Work out the finished part from the listing and answer in its coordinate system (mm). A direction names the side the tool comes from. Give positions to 0.01 mm unless a question says otherwise; leave off trailing zeros. Loops run counter-clockwise (first coordinate to the right, second up) from the corner with the lowest first, then second, coordinate; pieces in that order, holes last. Notation, with made-up numbers: M 77.5,30.5 L 89.5,30.5 A21 cw 89.5,40.5 Z; hole C 67.5,58.25 d6. An arc over 180 degrees is marked long. Use a Markdown table: item, result.
```python
from build123d import *

# Parameters (mm, degrees)
IZIM1_R                     = 5.4
IZIM1_R_2                   = 1.75
Y_KSEKLIK_EKSTR_ZYON1_DEPTH = 10.5
IZIM3_W                     = 5.5
IZIM3_H                     = 14
KES_EKSTR_ZYON1_DEPTH       = 34.5
KES_EKSTR_ZYON2_DEPTH       = 34.5
KES_EKSTR_ZYON2_DEPTH_BACK  = 34.5
IZIM5_W                     = 6.606601718
IZIM5_H                     = 5.5
KES_EKSTR_ZYON4_DEPTH       = 50.5
KES_EKSTR_ZYON5_DEPTH       = 5.5
Y_KSEKLIK_EKSTR_ZYON2_DEPTH = 8
RADYUS2_R                   = 8
RADYUS7_R                   = 4
IZIM9_W                     = 23
IZIM9_H                     = 13
KES_EKSTR_ZYON6_DEPTH       = 8.5
IZIM10_R                    = 1
KES_EKSTR_ZYON7_DEPTH       = 6
KES_EKSTR_ZYON8_DEPTH       = 4
IZIM12_R                    = 1.3
IZIM12_R_2                  = 2.5
KES_EKSTR_ZYON9_DEPTH       = 8
IZIM13_R                    = 2.5
Y_KSEKLIK_EKSTR_ZYON4_DEPTH = 8
IZIM14_R                    = 3.75
IZIM14_R_2                  = 1.5
KES_EKSTR_ZYON10_DEPTH      = 8
IZIM15_W                    = 10
IZIM15_H                    = 20
IZIM15_R                    = 1.5
KES_EKSTR_ZYON11_DEPTH      = 4
RADYUS10_R                  = 3
RADYUS11_R                  = 3
RADYUS12_R                  = 3
RADYUS13_R                  = 3


with BuildPart() as part:
    # Çizim1 → Yükseklik-Ekstrüzyon1 (new body)
    with BuildSketch(Plane.XY):
        with BuildLine():
            ThreePointArc((-10.23959488, -42.821815771), (-10.512642946, -42.272926126), (-10.606601718, -41.667115232))
            Line((-10.606601718, -41.667115232), (-10.606601718, -23.737818565))
            ThreePointArc((-10.606601718, -23.737818565), (-10.454360783, -22.972451701), (-10.02081528, -22.323605003))
            Line((-10.02081528, -22.323605003), (-4.585786438, -16.888576161))
            ThreePointArc((-4.585786438, -16.888576161), (-4.152240935, -16.239729463), (-4, -15.474362598))
            Line((-4, -15.474362598), (-4, -12.302789723))
            Line((-4, -12.302789723), (-4, 32.697210277))
            Line((-4, 32.697210277), (4, 32.697210277))
            Line((4, 32.697210277), (4, -8.302789723))
            ThreePointArc((4, -8.302789723), (5.171572875, -11.131216848), (8, -12.302789723))
            Line((8, -12.302789723), (15.171572875, -12.302789723))
            ThreePointArc((15.171572875, -12.302789723), (15.93693974, -12.455030658), (16.585786438, -12.888576161))
            Line((16.585786438, -12.888576161), (25.414213562, -21.717003285))
            ThreePointArc((25.414213562, -21.717003285), (26.06306026, -22.150548788), (26.828427125, -22.302789723))
            Line((26.828427125, -22.302789723), (30, -22.302789723))
            ThreePointArc((30, -22.302789723), (32.828427125, -23.474362598), (34, -26.302789723))
            Line((34, -26.302789723), (34, -38.302789723))
            ThreePointArc((34, -38.302789723), (32.828427125, -41.131216848), (30, -42.302789723))
            Line((30, -42.302789723), (26.317150887, -42.302789723))
            ThreePointArc((26.317150887, -42.302789723), (25.340138032, -42.557669131), (24.612145635, -43.257343842))
            Line((24.612145635, -43.257343842), (16.877945687, -55.870958544))
            ThreePointArc((16.877945687, -55.870958544), (15.785957092, -56.920470611), (14.320437809, -57.302789723))
            Line((14.320437809, -57.302789723), (1.552914271, -57.302789723))
            ThreePointArc((1.552914271, -57.302789723), (0.17381174, -56.967011225), (-0.896575472, -56.03484053))
            Line((-0.896575472, -56.03484053), (-10.23959488, -42.821815771))
        make_face()
        with Locations((23.814213562, -32.302789723)):
            Circle(IZIM1_R, mode=Mode.SUBTRACT)
        with Locations((-5.606601718, -32.302789723)):
            Circle(IZIM1_R_2, mode=Mode.SUBTRACT)
        with Locations((13, -52.302789723)):
            Circle(IZIM1_R_2, mode=Mode.SUBTRACT)
        with Locations((3, -52.302789723)):
            Circle(IZIM1_R_2, mode=Mode.SUBTRACT)
    extrude(amount=Y_KSEKLIK_EKSTR_ZYON1_DEPTH)

    # Çizim3 → Kes-Ekstrüzyon1 (cut)
    with BuildSketch(Plane(origin=(4, 0, 0), x_dir=(0, 0, -1), z_dir=(1, 0, 0))):
        with Locations((-2.75, -15.302789723)):
            Rectangle(IZIM3_W, IZIM3_H)
    extrude(amount=KES_EKSTR_ZYON1_DEPTH, mode=Mode.SUBTRACT)

    # Çizim4 → Kes-Ekstrüzyon2 (cut, two sides)
    with BuildSketch(Plane(origin=(0, 0, 0), x_dir=(0, 0, -1), z_dir=(1, 0, 0))) as kes_ekstr_zyon2_sk:
        Polygon((-5.5, -42.821815771), (-5.5, -42.302789723), (0, -42.302789723), (0, -42.821815771), (0, -57.302789723), (-5.5, -57.302789723), align=None)
    extrude(amount=KES_EKSTR_ZYON2_DEPTH, mode=Mode.SUBTRACT)
    extrude(kes_ekstr_zyon2_sk.sketch, amount=-KES_EKSTR_ZYON2_DEPTH_BACK, mode=Mode.SUBTRACT)

    # Çizim5 → Kes-Ekstrüzyon4 (cut)
    with BuildSketch(Plane(origin=(0, 0, 0), x_dir=(1, 0, 0), z_dir=(0, 1, 0))):
        with Locations((-7.303300859, -2.75)):
            Rectangle(IZIM5_W, IZIM5_H)
    extrude(amount=-KES_EKSTR_ZYON4_DEPTH, mode=Mode.SUBTRACT)

    # Çizim7 → Kes-Ekstrüzyon5 (cut)
    with BuildSketch(Plane.XY):
        with BuildLine():
            Line((-4.606601718, -22.909391441), (-10.606601718, -22.909391441))
            Line((-10.606601718, -22.909391441), (-12.80795169, -22.909391441))
            Line((-12.80795169, -22.909391441), (-12.80795169, -45.448338302))
            Line((-12.80795169, -45.448338302), (4.393398282, -45.448338302))
            Line((4.393398282, -45.448338302), (4.393398282, -42.302789723))
            ThreePointArc((4.393398282, -42.302789723), (0.857864376, -40.838323629), (-0.606601718, -37.302789723))
            Line((-0.606601718, -37.302789723), (-0.606601718, -26.909391441))
            ThreePointArc((-0.606601718, -26.909391441), (-1.778174593, -24.080964316), (-4.606601718, -22.909391441))
        make_face()
    extrude(amount=KES_EKSTR_ZYON5_DEPTH, mode=Mode.SUBTRACT)

    # Çizim8 → Yükseklik-Ekstrüzyon2 (add)
    with BuildSketch(Plane(origin=(4, 0, 0), x_dir=(0, 0, -1), z_dir=(1, 0, 0))):
        with BuildLine():
            Line((-10.5, 32.697210277), (9.5, 32.697210277))
            ThreePointArc((9.5, 32.697210277), (15.156854249, 30.354064527), (17.5, 24.697210277))
            Line((17.5, 24.697210277), (17.5, -1.336305369))
            Line((17.5, -1.336305369), (17.5, -1.489081224))
            ThreePointArc((17.5, -1.489081224), (16.89103626, -4.550548683), (15.156854249, -7.145935473))
            Line((15.156854249, -7.145935473), (0, -22.302789723))
            Line((0, -22.302789723), (-10.5, -22.302789723))
            Line((-10.5, -22.302789723), (-10.5, 32.697210277))
        make_face()
    extrude(amount=-Y_KSEKLIK_EKSTR_ZYON2_DEPTH)

    # Radyus2
    radyus2_edges = [part.edges().sort_by_distance(p)[0] for p in [
        (0, 32.697210277, 10.5),
    ]]
    fillet(radyus2_edges, radius=RADYUS2_R)

    # Radyus7
    radyus7_edges = [part.edges().sort_by_distance(p)[0] for p in [
        (4, -22.302789723, 2.75),
    ]]
    fillet(radyus7_edges, radius=RADYUS7_R)

    # Çizim9 → Kes-Ekstrüzyon6 (cut)
    with BuildSketch(Plane.XY):
        with Locations((18.5, -32.302789723)):
            Rectangle(IZIM9_W, IZIM9_H)
    extrude(amount=KES_EKSTR_ZYON6_DEPTH, mode=Mode.SUBTRACT)

    # Çizim10 → Kes-Ekstrüzyon7 (cut)
    with BuildSketch(Plane.XY):
        with Locations((32, -32.302789723)):
            Circle(IZIM10_R)
        with Locations((5, -32.302789723)):
            Circle(IZIM10_R)
    extrude(amount=KES_EKSTR_ZYON7_DEPTH, mode=Mode.SUBTRACT)

    # Çizim11 → Kes-Ekstrüzyon8 (cut)
    with BuildSketch(Plane.ZY.offset(4)):
        with BuildLine():
            Line((-6.5, 14.197210277), (-6.5, 23.197210277))
            ThreePointArc((-6.5, 23.197210277), (-3.5, 26.197210277), (-0.5, 23.197210277))
            Line((-0.5, 23.197210277), (-0.5, 14.197210277))
            ThreePointArc((-0.5, 14.197210277), (-3.5, 11.197210277), (-6.5, 14.197210277))
        make_face()
    extrude(amount=-KES_EKSTR_ZYON8_DEPTH, mode=Mode.SUBTRACT)

    # Çizim12 → Kes-Ekstrüzyon9 (cut)
    with BuildSketch(Plane.ZY.offset(4)):
        with Locations((-3.5, 23.197210277)):
            Circle(IZIM12_R)
        with Locations((-3.5, 14.197210277)):
            Circle(IZIM12_R)
        with Locations((-3.5, 18.697210277)):
            Circle(IZIM12_R_2)
    extrude(amount=-KES_EKSTR_ZYON9_DEPTH, mode=Mode.SUBTRACT)

    # Çizim13 → Yükseklik-Ekstrüzyon4 (add)
    with BuildSketch(Plane(origin=(4, 0, 0), x_dir=(0, 0, -1), z_dir=(1, 0, 0))):
        Polygon((-4.189470597, 27.846393302), (11.202467705, 28.228364897), (11.683763176, 8.834068822), (-4.189470597, 8.440153234), align=None)
        with Locations((3.5, 18.697210277)):
            Circle(IZIM13_R, mode=Mode.SUBTRACT)
    extrude(amount=-Y_KSEKLIK_EKSTR_ZYON4_DEPTH)

    # Çizim14 → Kes-Ekstrüzyon10 (cut)
    with BuildSketch(Plane(origin=(4, 0, 0), x_dir=(0, 0, -1), z_dir=(1, 0, 0))):
        with Locations((3.5, 19.50634608)):
            Circle(IZIM14_R)
        with Locations((3.5, 12.25634608)):
            Circle(IZIM14_R_2)
        with Locations((3.5, 26.75634608)):
            Circle(IZIM14_R_2)
    extrude(amount=-KES_EKSTR_ZYON10_DEPTH, mode=Mode.SUBTRACT)

    # Çizim15 → Kes-Ekstrüzyon11 (cut)
    with BuildSketch(Plane.ZY.offset(4)):
        with Locations((-3.5, 19.50634608)):
            Rectangle(IZIM15_W, IZIM15_H)
        with Locations((-3.5, 26.75634608)):
            Circle(IZIM15_R, mode=Mode.SUBTRACT)
    extrude(amount=-KES_EKSTR_ZYON11_DEPTH, mode=Mode.SUBTRACT)

    # Radyus10
    radyus10_edges = [part.edges().sort_by_distance(p)[0] for p in [
        (-2, 29.50634608, 1.5),
    ]]
    fillet(radyus10_edges, radius=RADYUS10_R)

    # Radyus11
    radyus11_edges = [part.edges().sort_by_distance(p)[0] for p in [
        (-2, 9.50634608, -8.5),
    ]]
    fillet(radyus11_edges, radius=RADYUS11_R)

    # Radyus12
    radyus12_edges = [part.edges().sort_by_distance(p)[0] for p in [
        (-2, 29.50634608, -8.5),
    ]]
    fillet(radyus12_edges, radius=RADYUS12_R)

    # Radyus13
    radyus13_edges = [part.edges().sort_by_distance(p)[0] for p in [
        (-2, 9.50634608, 1.5),
    ]]
    fillet(radyus13_edges, radius=RADYUS13_R)


solid = part.part
```
(1) Given P1, Ø10, axis at x = 18, y = -36, coming from the -Z side; P2, Ø0.6, axis at x = 32, y = -32.5, coming from the -Z side; P3, Ø2.5, axis at y = -32.5, z = 4, coming from the -X side; P4, Ø10, axis at x = -2.5, z = 7.5, coming from the +Y side, each flat-ended and moving along its own axis, determine where each tip first touches the part or whether it passes through.
Entries:
| item | result |
|---|---|
| P1 | stops at z = 0 |
| P2 | stops at z = 6 |
| P3 | stops at x = -0.61 |
| P4 | stops at y = 32.7 |
(2) A cutting plane is placed at D-D (z = -13.75). Write down the section's boundary in (x, y).
Entries:
| item | result |
|---|---|
| outline | M -4,-8.55 L 4,-8.55 L 4,31.47 L -4,31.47 Z |
(3) The mould has two halves that part along X. Classify faces 6 (the cylindrical face through (-1.972, 10.362, 0.598)), 7 (the flat face through (-0.607, -32, 3)), 8 (the cylindrical face through (3.9, -50.8, 8)): released by +X, released by -X, zero draft, split by the parting line, or undercut.
Entries:
| item | result |
|---|---|
| face 6 | zero draft |
| face 7 | released by -X |
| face 8 | undercut |
(4) Consider probe 1 along Y at (x, z) = (3.25, -3.5); probe 2 along Z at (x, y) = (9.5, -38); probe 3 along Z at (x, y) = (31, -34). Determine where each line is inside the solid, lowest interval first. Write a range as [from, to].
Entries:
| item | result |
|---|---|
| probe 1 | y = [-18.8, 10.76], [13.76, 15.76], [23.26, 25.26], [28.26, 32.7] |
| probe 2 | z = [8.5, 10.5] |
| probe 3 | z = [0, 10.5] |
(5) Which of the six approach directions +Z, -Z, +X, -X, +Y, -Y give full straight-line access (tool end or side, diameter ignored) to faces 1 (the cylindrical face through (5.14, -21.1, 1.74)), 2 (the cylindrical face through (0.06, 30.29, 8.22)), 3 (the cylindrical face through (15.805, -56.91, 7.965)), 4 (the cylindrical face through (-1.97, 28.65, 0.6)), 5 (the cylindrical face through (31.78, -33.28, 2.96))?
Entries:
| item | result |
|---|---|
| face 1 | -Z, +X, +Y |
| face 2 | +Z, +X, -X, +Y |
| face 3 | +Z, -Z, +X, -Y |
| face 4 | -X |
| face 5 | -Z |
(6) A cutting plane is placed at A-A (x = 13). Write down the section's boundary in (y, z).
Entries:
| item | result |
|---|---|
| outline | M -57.3,5.5 L -54.05,5.5 L -54.05,10.5 L -57.3,10.5 Z; M -50.55,5.5 L -42.3,5.5 L -42.3,0 L -38.8,0 L -38.8,8.5 L -25.8,8.5 L -25.8,0 L -22.3,0 L -22.3,5.5 L -12.3,5.5 L -12.3,10.5 L -50.55,10.5 Z |
(7) A cutting plane is placed at B-B (x = -2). Write down the section's boundary in (y, z), and give its area (3 significant figures).
Entries:
| item | result |
|---|---|
| outline | M -54.47,5.5 L -23.88,5.5 L -23.88,0 L -22.3,0 L -7.15,-15.16 A8 ccw -1.49,-17.5 L 24.7,-17.5 A8 ccw 32.7,-9.5 L 32.7,2.5 A8 ccw 24.7,10.5 L -54.47,10.5 Z; hole M 9.51,-5.5 A3 ccw 12.51,-8.5 L 26.51,-8.5 A3 ccw 29.51,-5.5 L 29.51,-1.5 A3 ccw 26.51,1.5 L 12.51,1.5 A3 ccw 9.51,-1.5 Z |
| area | 1,340 mm² |
(8) A cutting plane is placed at C-C (y = 6.5). Write down the section's boundary in (x, z).
Entries:
| item | result |
|---|---|
| outline | M -4,-17.5 L 4,-17.5 L 4,10.5 L -4,10.5 Z |
